```python
from build123d import *

# Parameters (mm, degrees)
F1_DEPTH = 12.7
F0_W     = 101.6
F0_H     = 3.175
F2_DEPTH = 152.4
F3_DEPTH = 50.8
F4_W     = 101.6
F4_H     = 3.175
F5_DEPTH = 50.8
F6_W     = 38.1
F6_H     = 38.1
F7_DEPTH = 25.4


with BuildPart() as f1:
    # F0 (on Top) → F1 (new body)
    with BuildSketch(Plane.XY):
        with BuildLine():
            Line((41.043708, 6.35), (-60.556292, 6.35))
            ThreePointArc((-60.556292, 6.35), (-66.906292, 0), (-60.556292, -6.35))
            Line((-60.556292, -6.35), (41.043708, -6.35))
            ThreePointArc((41.043708, -6.35), (47.393708, 0), (41.043708, 6.35))
        make_face()
    extrude(amount=F1_DEPTH)

    # F0 (on Top) → F2 (join)
    with BuildSketch(Plane.XY):
        with BuildLine():
            ThreePointArc((-60.556292, -6.35), (-66.906292, 0), (-60.556292, 6.35))
            Line((-60.556292, 6.35), (41.043708, 6.35))
            ThreePointArc((41.043708, 6.35), (47.393708, 0), (41.043708, -6.35))
            Line((41.043708, -6.35), (41.043708, -9.525))
            ThreePointArc((41.043708, -9.525), (50.568708, 0), (41.043708, 9.525))
            Line((41.043708, 9.525), (-60.556292, 9.525))
            ThreePointArc((-60.556292, 9.525), (-70.081292, 0), (-60.556292, -9.525))
            Line((-60.556292, -9.525), (-60.556292, -6.35))
        make_face()
        with Locations((-9.756292, -7.9375)):
            Rectangle(F0_W, F0_H)
    extrude(amount=F2_DEPTH)

    # F0 (on Top) → F3 (join)
    with BuildSketch(Plane.XY):
        with Locations((-9.756292, -7.9375)):
            Rectangle(F0_W, F0_H)
    extrude(amount=F3_DEPTH)

    # F4 (on face) → F5 (join)
    with BuildSketch(Plane.XY.offset(152.4)):
        with Locations((-9.756292, 7.9375)):
            Rectangle(F4_W, F4_H)
    extrude(amount=F5_DEPTH)

    # F6 (on face) → F7 (cut)
    with BuildSketch(Plane(origin=(0, 9.525, 0), x_dir=(-1, 0, 0), z_dir=(0, 1, 0))):
        with Locations((9.756292, 177.8)):
            Rectangle(F6_W, F6_H)
    extrude(amount=-F7_DEPTH, mode=Mode.SUBTRACT)


solid = f1.part
```
Model file for the job. Use its own axes, mm. A direction names the side the tool comes from. Round coordinates to 2 decimals unless told otherwise and drop trailing zeros. Write each loop counter-clockwise with the first axis right and the second up, starting at its lowest first coordinate (ties: lowest second). Pieces come first, ordered by that corner, then holes. Notation, with made-up numbers: (-7, -9) - (26, -9) arc R11 ccw to (26, 3) - close; hole circle Ø4 at (85, -39.5). An arc over 180 degrees is marked (long way). One line per item, written item: value.
(1) Cut at B-B, the plane x = 12. Give the cut face in (y, z) (3 decimals), plus the area to 3 significant figures.
Values follow:
outline: (-9.525, 0) - (9.525, 0) - (9.525, 203.2) - (6.35, 203.2) - (6.35, 12.7) - (-6.35, 12.7) - (-6.35, 152.4) - (-9.525, 152.4) - close
area: 1,290 mm²
(2) Two-plate mould, pull along X, no slides. Class faces 3 (the cylindrical face through (-70.08, 0.21, 75.13)), 4 (the flat face through (-11, 0, 0)), 5 (the cylindrical face through (47.392, 0.14, 81.572)): pulls with the +X half, pulls with the -X half, needs draft (parallel to the pull), parting line crosses it, or undercut.
Values follow:
face 3: pulls with the -X half
face 4: needs draft
face 5: undercut
(3) Drop flat-ended pins along their axis: P1, Ø3, axis at x = -40, y = 3, coming from the +Z side; P2, Ø1, axis at y = 8.5, z = 187, coming from the -X side; P3, Ø1, axis at y = 7.5, z = 189.5, coming from the +X side. Give the stop position or say it passes through.
Values follow:
P1: stops at z = 12.7
P2: stops at x = -60.56
P3: stops at x = 41.04
(4) Cut at A-A, the plane z = 169. Give the cut face in (x, y) (3 decimals).
Values follow:
outline: (-60.556, 6.35) - (-28.806, 6.35) - (-28.806, 9.525) - (-60.556, 9.525) - close; (9.294, 6.35) - (41.044, 6.35) - (41.044, 9.525) - (9.294, 9.525) - close
(5) Cut at D-D, the plane y = 0. Give the cut face in (x, z), plus the area to 3 significant figures.
Values follow:
outline: (-70.08, 0) - (50.57, 0) - (50.57, 152.4) - (47.39, 152.4) - (47.39, 12.7) - (-66.91, 12.7) - (-66.91, 152.4) - (-70.08, 152.4) - close
area: 2,420 mm²
(6) Wall check: probe 1 along Y at (x, z) = (-17, 99) (3 decimals); probe 2 along X at (y, z) = (-0.5, 86); probe 3 along Z at (x, y) = (-20, 7.25). Give the ranges that are in metal, low to high.
Values follow:
probe 1: y = -9.525 to -6.35, 6.35 to 9.525
probe 2: x = -70.07 to -66.89, 47.37 to 50.56
probe 3: z = 0 to 158.75, 196.85 to 203.2
(7) Cut at C-C, the plane z = 99. Give the cut face in (x, y) (3 decimals).
Values follow:
outline: (-60.556, -9.525) - (41.044, -9.525) arc R9.525 ccw to (41.044, 9.525) - (-60.556, 9.525) arc R9.525 ccw to start; hole (-60.556, -6.35) - (41.044, -6.35) arc R6.35 ccw to (41.044, 6.35) - (-60.556, 6.35) arc R6.35 ccw to start
(8) 3-axis set-ups, long thin cutter, end or side, ignore diameter. For faces 1 (the flat face through (-11, 0, 12.7)), 2 (the flat face through (-10, 9.525, 100)): which of +Z, -Z, +X, -X, +Y, -Y reach the whole face in a straight line?
Values follow:
face 1: +Z
face 2: +Z, -Z, +X, -X, +Y
